```python
from build123d import *

# Parameters (mm, degrees)
SKETCH_1_R      = 2.1
SKETCH_1_R_2    = 1.6
SKETCH_1_W      = 20
SKETCH_1_H      = 41
EXTRUDE_1_DEPTH = 1.6


with BuildPart() as part:
    # 草图1 → 凸台-拉伸1 (new body)
    with BuildSketch(Plane.XY):
        Polygon((-30, 46.5), (-28, 48.5), (28, 48.5), (30, 46.5), (30, -46.5), (28, -48.5), (-28, -48.5), (-30, -46.5), align=None)
        with Locations((-11.75, 38.5)):
            Circle(SKETCH_1_R, mode=Mode.SUBTRACT)
        with Locations((-5, 23.7)):
            Circle(SKETCH_1_R_2, mode=Mode.SUBTRACT)
        with Locations(Location((-5, -23.7, 0), (0, 0, 180))):
            Circle(SKETCH_1_R_2, mode=Mode.SUBTRACT)
        with Locations(Location((-11.75, -38.5, 0), (0, 0, 180))):
            Circle(SKETCH_1_R, mode=Mode.SUBTRACT)
        with Locations((11.75, -38.5)):
            Circle(SKETCH_1_R, mode=Mode.SUBTRACT)
        with Locations((5, -23.7)):
            Circle(SKETCH_1_R_2, mode=Mode.SUBTRACT)
        with Locations(Location((5, 23.7, 0), (0, 0, 180))):
            Circle(SKETCH_1_R_2, mode=Mode.SUBTRACT)
        with Locations(Location((11.75, 38.5, 0), (0, 0, 180))):
            Circle(SKETCH_1_R, mode=Mode.SUBTRACT)
        with BuildLine():
            Line((-18.12722641, 10), (-18.12722641, -10))
            ThreePointArc((-18.12722641, -10), (-16.12722641, -12), (-14.12722641, -10))
            Line((-14.12722641, -10), (-14.12722641, 10))
            ThreePointArc((-14.12722641, 10), (-16.12722641, 12), (-18.12722641, 10))
        make_face(mode=Mode.SUBTRACT)
        Rectangle(SKETCH_1_W, SKETCH_1_H, mode=Mode.SUBTRACT)
        with BuildLine():
            Line((18.12722641, 10), (18.12722641, -10))
            ThreePointArc((18.12722641, -10), (16.12722641, -12), (14.12722641, -10))
            Line((14.12722641, -10), (14.12722641, 10))
            ThreePointArc((14.12722641, 10), (16.12722641, 12), (18.12722641, 10))
        make_face(mode=Mode.SUBTRACT)
    extrude(amount=EXTRUDE_1_DEPTH)


solid = part.part
```
Can you work these out from the model? Positions are in its coordinate system, mm. A direction names the side the tool comes from. Give positions to 0.01 mm unless a question says otherwise; leave off trailing zeros. Order: outer loops, then holes, each group sorted by start corner. A loop starts at its lowest first (then second) coordinate and runs counter-clockwise, first axis right, second up. Notation, with made-up numbers: (-13.5, 64) - (35.5, 64) arc R19 ccw to (35.5, 78) - close; hole circle Ø4 at (40, -12). An arc over 180 degrees is marked (long way). Use a Markdown table: item, result. Add a question column.
Q1. On a 3-axis mill with a long thin cutter (end or side, diameter ignored), from which of +Z, -Z, +X, -X, +Y, -Y can I reach the whole of each face in a straight line? I mean faces 5 (the flat face through (29, 47.5, 0.8)), 6 (the cylindrical face through (16.1, 12, 0.8)). Say none if no direction works.
Q2. If we mould it in two halves opening along X, with no side actions, what happens to faces 1 (the cylindrical face through (-16.1, 12, 0.8)), 2 (the cylindrical face through (6.27, 24.67, 0.79)), 3 (the flat face through (13.8, 0.7, 0)), 4 (the flat face through (29, -47.5, 0.8))? For each: released by +X, released by -X, zero draft, split by the parting line, or undercut.
Q3. If we section it at D-D on x = 11.75: Write out the boundary of the cut face in (y, z), plus the area to 3 significant figures.
Q4. If we section it at A-A on x = -5: Write out the boundary of the cut face in (y, z), plus the area to 3 significant figures.
Q5. If we section it at C-C on z = 0.85: Count the separate pieces of the cut face and the enclosed holes in it, plus the area to 3 significant figures.
Q6. If we section it at B-B on y = 19: Write out the boundary of the cut face in (x, z), plus the area to 3 significant figures.
Q7. I'm going to push a flat-ended pin straight in: pin 1 (2.5 mm diameter, centred on x = -5, y = -23.7, fed in from -Z). Where does the tip first touch, or does it pass through?
Q8. Please list where these lines run through material, in increasing order: line 1 along Y through (x, z) = (5, 0.85); line 2 along Y through (x, z) = (-11.75, 1.05); line 3 along Y through (x, z) = (-8, 1.2).
Answers follow:
| question | item | result |
|---|---|---|
| 1 | face 5 | +Z, -Z, +X, +Y |
| 1 | face 6 | +Z, -Z |
| 2 | face 1 | undercut |
| 2 | face 2 | undercut |
| 2 | face 3 | zero draft |
| 2 | face 4 | released by +X |
| 3 | outline | (-48.5, 0) - (-40.6, 0) - (-40.6, 1.6) - (-48.5, 1.6) - close; (-36.4, 0) - (36.4, 0) - (36.4, 1.6) - (-36.4, 1.6) - close; (40.6, 0) - (48.5, 0) - (48.5, 1.6) - (40.6, 1.6) - close |
| 3 | area | 142 mm^2 |
| 4 | outline | (-48.5, 0) - (-25.3, 0) - (-25.3, 1.6) - (-48.5, 1.6) - close; (-22.1, 0) - (-20.5, 0) - (-20.5, 1.6) - (-22.1, 1.6) - close; (20.5, 0) - (22.1, 0) - (22.1, 1.6) - (20.5, 1.6) - close; (25.3, 0) - (48.5, 0) - (48.5, 1.6) - (25.3, 1.6) - close |
| 4 | area | 79.4 mm^2 |
| 5 | separate pieces | 1 |
| 5 | enclosed holes | 11 |
| 5 | area | 4,720 mm^2 |
| 6 | outline | (-30, 0) - (-10, 0) - (-10, 1.6) - (-30, 1.6) - close; (10, 0) - (30, 0) - (30, 1.6) - (10, 1.6) - close |
| 6 | area | 64.0 mm^2 |
| 7 | pin 1 | passes through |
| 8 | line 1 | y = -48.5 to -25.3, -22.1 to -20.5, 20.5 to 22.1, 25.3 to 48.5 |
| 8 | line 2 | y = -48.5 to -40.6, -36.4 to 36.4, 40.6 to 48.5 |
| 8 | line 3 | y = -48.5 to -20.5, 20.5 to 48.5 |
